```python
from build123d import *

# Parameters (mm, degrees)
SKETCH1_W           = 36
SKETCH1_H           = 36
BOSS_EXTRUDE1_DEPTH = 1.5
SKETCH2_R           = 1.5
CUT_EXTRUDE1_DEPTH  = 26.5
SKETCH5_W           = 5.4
SKETCH5_H           = 22
BOSS_EXTRUDE4_DEPTH = 4.5
SKETCH6_W           = 16
SKETCH6_H           = 16
BOSS_EXTRUDE5_DEPTH = 5
SKETCH7_R           = 14
BOSS_EXTRUDE6_DEPTH = 31


with BuildPart() as part:
    # Sketch1 → Boss-Extrude1 (new body)
    with BuildSketch(Plane(origin=(0, 0, 0), x_dir=(1, 0, 0), z_dir=(0, 1, 0))):
        Rectangle(SKETCH1_W, SKETCH1_H)
    extrude(amount=BOSS_EXTRUDE1_DEPTH)

    # Sketch2 → Cut-Extrude1 (cut, through all)
    with BuildSketch(Plane(origin=(0, 1.5, 0), x_dir=(1, 0, 0), z_dir=(0, 1, 0))):
        with Locations(Location((14, 14, 0), (0, 0, 270))):
            Circle(SKETCH2_R)
        with Locations(Location((14, -14, 0), (0, 0, 270))):
            Circle(SKETCH2_R)
        with Locations(Location((-14, -14, 0), (0, 0, 270))):
            Circle(SKETCH2_R)
        with Locations(Location((-14, 14, 0), (0, 0, 270))):
            Circle(SKETCH2_R)
    extrude(amount=-CUT_EXTRUDE1_DEPTH, mode=Mode.SUBTRACT)

    # Sketch5 → Boss-Extrude4 (add)
    with BuildSketch(Plane(origin=(0, 1.5, 0), x_dir=(1, 0, 0), z_dir=(0, 1, 0))):
        with Locations((15.3, 0)):
            Rectangle(SKETCH5_W, SKETCH5_H)
    extrude(amount=BOSS_EXTRUDE4_DEPTH)

    # Sketch6 → Boss-Extrude5 (add)
    with BuildSketch(Plane(origin=(0, 1.5, 0), x_dir=(1, 0, 0), z_dir=(0, 1, 0))):
        Rectangle(SKETCH6_W, SKETCH6_H)
    extrude(amount=BOSS_EXTRUDE5_DEPTH)

    # Sketch7 → Boss-Extrude6 (add)
    with BuildSketch(Plane(origin=(0, 6.5, 0), x_dir=(1, 0, 0), z_dir=(0, 1, 0))):
        with Locations(Location((0, 0, 0), (0, 0, 270))):
            Circle(SKETCH7_R)
    extrude(amount=BOSS_EXTRUDE6_DEPTH)


solid = part.part
```
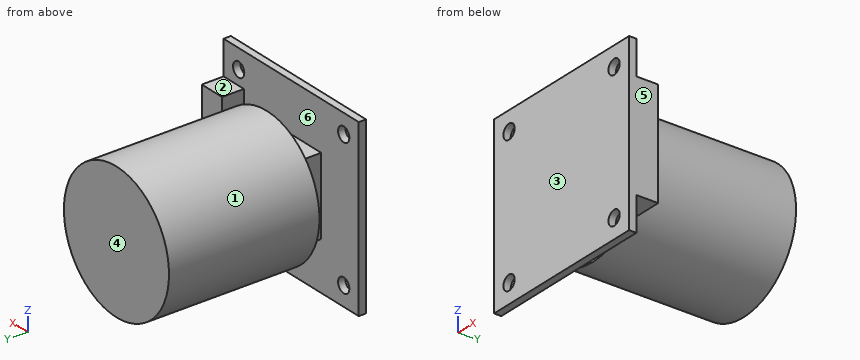
The model under review builds one solid part; all positions refer to its coordinate system, in mm. Face numbers are marked on the shaded views. A direction names the side the tool comes from. Coordinates: 2 decimals unless noted, no trailing zeros. Loops run counter-clockwise (first coordinate to the right, second up) from the corner with the lowest first, then second, coordinate; pieces in that order, holes last. Notation, with made-up numbers: (62.25, -16.5) -> (75.25, -16.5) arc R16 cw to (75.25, 4.5) -> close; hole circle Ø9 at (65.25, 14.25). An arc over 180 degrees is marked (long way). Answer as CSV lines item,"result".
Item 1: Machinability: for the marked faces 1, 2 and 3, which of the approach directions +Z, -Z, +X, -X, +Y, -Y give a long, thin tool a straight path to every point of the face, cutting with its end or side? Answer none if there is none.
Results below:
face 1,"+Y"
face 2,"+Z, +X, -X, +Y"
face 3,"+Z, -Z, +X, -X, -Y"
Item 2: Draft analysis for pull direction Y (two halves, no side actions). For the marked faces 4, 5 and 6, state which applies: +Y half, -Y half, draft (parallel to the pull), parting line (faces both ways), or undercut.
Results below:
face 4,"+Y half"
face 5,"draft"
face 6,"undercut"
Item 3: Take a section at C-C, the plane x = 0. State the section outline as (y, z) points.
Results below:
outline,"(0, -18) -> (1.5, -18) -> (1.5, -8) -> (6.5, -8) -> (6.5, -14) -> (37.5, -14) -> (37.5, 14) -> (6.5, 14) -> (6.5, 8) -> (1.5, 8) -> (1.5, 18) -> (0, 18) -> close"
Item 4: Insertion check: pin 1 (8 mm diameter, centred on x = -10, y = 10, fed in from +Z); pin 2 (1.5 mm diameter, centred on x = 9, y = 29.5, fed in from +Z); pin 3 (10 mm diameter, centred on y = 12.5, z = -13.5, fed in from -X). Each pin has a flat end and moves straight along its axis. Give the tip position at first contact, or say it passes through.
Results below:
pin 1,"stops at z = 12.65"
pin 2,"stops at z = 11.31"
pin 3,"stops at x = -11.12"
Item 5: For L1, parallel to X at y = 1, z = -14; L2, parallel to Y at x = -9.5, z = 0; L3, parallel to X at y = 4.5, z = 2.5, list the stretches that pass through material, from the lowest coordinate up.
Results below:
L1,"x = -18 to -15.5, -12.5 to 12.5, 15.5 to 18"
L2,"y = 0 to 1.5, 6.5 to 37.5"
L3,"x = -8 to 8, 12.6 to 18"
Item 6: Take a section at B-B, the plane z = 0. State the section outline as (x, y) points, and give its area (3 significant figures).
Results below:
outline,"(-18, 0) -> (18, 0) -> (18, 6) -> (12.6, 6) -> (12.6, 1.5) -> (8, 1.5) -> (8, 6.5) -> (14, 6.5) -> (14, 37.5) -> (-14, 37.5) -> (-14, 6.5) -> (-8, 6.5) -> (-8, 1.5) -> (-18, 1.5) -> close"
area,"1,030 mm2"
Item 7: Take a section at A-A, the plane y = 4. State the section outline as (x, z) points, and give its area (3 significant figures).
Results below:
outline,"(-8, -8) -> (8, -8) -> (8, 8) -> (-8, 8) -> close; (12.6, -11) -> (18, -11) -> (18, 11) -> (12.6, 11) -> close"
area,"375 mm2"
Item 8: Take a section at D-D, the plane x = 6. State the section outline as (y, z) points, and give its area (3 significant figures).
Results below:
outline,"(0, -18) -> (1.5, -18) -> (1.5, -8) -> (6.5, -8) -> (6.5, -12.65) -> (37.5, -12.65) -> (37.5, 12.65) -> (6.5, 12.65) -> (6.5, 8) -> (1.5, 8) -> (1.5, 18) -> (0, 18) -> close"
area,"918 mm2"
